```python
from build123d import *

# Parameters (mm, degrees)
F0_R     = 4.2
F1_DEPTH = 5
F2_SIZE  = 4.7


# Not quite as in the source:
# - a feature names something its author has since deleted; it is built from what else it names


with BuildPart() as f1:
    # F0 (on Front) → F1 (new body)
    with BuildSketch(Plane.XZ):
        with BuildLine():
            Line((58, 20), (-18, 20))
            ThreePointArc((-18, 20), (-19.4142135624, 19.4142135624), (-20, 18))
            Line((-20, 18), (-20, -18))
            ThreePointArc((-20, -18), (-19.4142135624, -19.4142135624), (-18, -20))
            Line((-18, -20), (58, -20))
            ThreePointArc((58, -20), (59.4142135624, -19.4142135624), (60, -18))
            Line((60, -18), (60, 18))
            ThreePointArc((60, 18), (59.4142135624, 19.4142135624), (58, 20))
        make_face()
        Circle(F0_R, mode=Mode.SUBTRACT)
        with Locations((40, 0)):
            Circle(F0_R, mode=Mode.SUBTRACT)
    extrude(amount=F1_DEPTH)

    # F2
    f2_edges = [f1.edges().sort_by_distance(p)[0] for p in [
        (-4.2, -5, 0),
        (35.8, -5, 0),
    ]]
    chamfer(f2_edges, length=F2_SIZE)


solid = f1.part
```
CAD build for the part. Positions are in the model's coordinates, mm. Coordinates: 2 decimals unless noted, no trailing zeros. Order: outer loops, then holes, each group sorted by start corner. A loop starts at its lowest first (then second) coordinate and runs counter-clockwise, first axis right, second up. Notation, with made-up numbers: (22, -13.5) - (59, -13.5) arc R16 ccw to (59, -1.5) - close; hole circle Ø9 at (-13, 54.25). An arc over 180 degrees is marked (long way). Answer in a Markdown table with one row per item.
1. Pull direction Z, two halves, no side cores. Call faces 1 (the face through (-0.91, -0.15, -4.1)), 2 (the face through (-20, -2, 0)), 3 (the face through (35.51, -0.594, 0.198)), 4 (the face through (-19.4, -2.46, 19.43)): +Z half, -Z half, draft (parallel to the pull), parting line (faces both ways), or undercut.
Answer:
| item | result |
|---|---|
| face 1 | undercut |
| face 2 | draft |
| face 3 | undercut |
| face 4 | +Z half |
2. Slice it at B-B, the plane x = 0. List the corners of the cut face in (y, z).
Answer:
| item | result |
|---|---|
| outline | (-5, -20) - (0, -20) - (0, -4.2) - (-0.3, -4.2) - (-5, -8.9) - close; (-5, 8.9) - (-0.3, 4.2) - (0, 4.2) - (0, 20) - (-5, 20) - close |
3. Drill centre lines: L1, parallel to Z at x = 40, y = -0.2; L2, parallel to X at y = -1.7, z = 3; L3, parallel to X at y = -4.1, z = 2.5. Where is each one in solid material? Low to high. Write a range as from..to.
Answer:
| item | result |
|---|---|
| L1 | -20..-4.2, 4.2..20 |
| L2 | -20..-4.73, 4.73..35.27, 44.73..60 |
| L3 | -20..-7.6, 7.6..32.4, 47.6..60 |
4. Slice it at A-A, the plane y = -2.45. List the corners of the cut face in (x, z).
Answer:
| item | result |
|---|---|
| outline | (-20, -18) arc R2 ccw to (-18, -20) - (58, -20) arc R2 ccw to (60, -18) - (60, 18) arc R2 ccw to (58, 20) - (-18, 20) arc R2 ccw to (-20, 18) - close; hole circle Ø12.7 at (0, 0); hole circle Ø12.7 at (40, 0) |
5. Flat gauge pins, fed straight in: P1, Ø6.5, axis at x = 40, z = 0, coming from the +Y side; P2, Ø6, axis at x = 37.5, z = 0.5, coming from the -Y side. Where does each tip first touch, or does it go through?
Answer:
| item | result |
|---|---|
| P1 | through |
| P2 | y = -1.65 |
6. Slice it at C-C, the plane z = -3. Give the number of separate pieces and of enclosed holes in the cut face, then the cut area to 3 significant figures.
Answer:
| item | result |
|---|---|
| separate pieces | 3 |
| enclosed holes | 0 |
| area | 288 mm² |
